```python
from build123d import *

# Parameters (mm, degrees)
F1_DEPTH = 130
F2_R     = 5.5
F3_DEPTH = 25
F2_R_2   = 9.5
F4_DEPTH = 13
F6_D     = 6.8
F7_D     = 8.8


# Not quite as in the source:
# - a pattern or mirror of a feature is missing from the dataset's text; its kind, count and spacing are read off the source's solid


with BuildPart() as f1:
    # F0 (on Front) → F1 (new body, symmetric)
    with BuildSketch(Plane.XZ):
        Polygon((-50, 23), (-50, 0), (45, 0), (45, -5), (50, -5), (50, 23), align=None)
    extrude(amount=F1_DEPTH, both=True)

    # F2 (on face) → F3 (cut)
    with BuildSketch(Plane.XY.offset(23)):
        with Locations((-36, -109)):
            Circle(F2_R)
        with Locations((36, -109)):
            Circle(F2_R)
        with Locations((-36, -57)):
            Circle(F2_R)
        with Locations((36, -57)):
            Circle(F2_R)
    f3 = extrude(amount=-F3_DEPTH, mode=Mode.SUBTRACT)

    # F3_copies: F3 across plane
    add(f3.mirror(Plane.ZX), mode=Mode.SUBTRACT)

    # F2 (on face) → F4 (cut)
    with BuildSketch(Plane.XY.offset(23)):
        with Locations((-36, -109)):
            Circle(F2_R_2)
        with Locations((-36, -109)):
            Circle(F2_R, mode=Mode.SUBTRACT)
        with Locations((36, -109)):
            Circle(F2_R_2)
        with Locations((36, -109)):
            Circle(F2_R, mode=Mode.SUBTRACT)
        with Locations((36, -109)):
            Circle(F2_R)
        with Locations((-36, -57)):
            Circle(F2_R_2)
        with Locations((-36, -57)):
            Circle(F2_R, mode=Mode.SUBTRACT)
        with Locations((36, -57)):
            Circle(F2_R_2)
        with Locations((36, -57)):
            Circle(F2_R, mode=Mode.SUBTRACT)
        with Locations((36, -57)):
            Circle(F2_R)
    f4 = extrude(amount=-F4_DEPTH, mode=Mode.SUBTRACT)

    # F4_copies: F4 across plane
    add(f4.mirror(Plane.ZX), mode=Mode.SUBTRACT)

    # F6 (through all)
    with Locations(Plane.XY.offset(23)):
        with Locations((-19, -115), (19, -115), (-19, -45), (19, -45), (19, -5), (-19, -5)):
            Hole(F6_D / 2)

    # F7 (through all)
    with Locations(Plane.XY.offset(23)):
        with Locations((-41, 35), (41, 35), (41, 90), (-41, 90)):
            Hole(F7_D / 2)


solid = f1.part
```
Can you work these out from the model? Positions are in its coordinate system, mm. A direction names the side the tool comes from. Round coordinates to 2 decimals unless told otherwise and drop trailing zeros. Order: outer loops, then holes, each group sorted by start corner. A loop starts at its lowest first (then second) coordinate and runs counter-clockwise, first axis right, second up.
(1) I'm going to push flat-ended pins straight in: pin 1 (3 mm diameter, centred on x = -0.5, y = -7.5, fed in from -Z); pin 2 (11.5 mm diameter, centred on x = -36, y = -57, fed in from +Z); pin 3 (4 mm diameter, centred on y = 111.5, z = -3, fed in from -X). Where does each tip first touch, or does it pass through?
Results are:
pin 1: stops at z = 0
pin 2: stops at z = 10
pin 3: stops at x = 45
(2) On a 3-axis mill with a long thin cutter (end or side, diameter ignored), from which of +Z, -Z, +X, -X, +Y, -Y can I reach the whole of each face in a straight line? I mean faces 5 (the face through (19.44, -41.63, 11.34)), 6 (the face through (-26.939, 106.146, 16.591)). Say none if no direction works.
Results are:
face 5: +Z, -Z
face 6: +Z
(3) If I drill on L1, parallel to Y at x = -35, z = 18; L2, parallel to Y at x = -36, z = 3.75; L3, parallel to Y at x = 19, z = 6, over which ranges is the centre line in solid material (lowest first)?
Results are:
L1: y = -130 to -118.45, -99.55 to -66.45, -47.55 to 47.55, 66.45 to 99.55, 118.45 to 130
L2: y = -130 to -114.5, -103.5 to -62.5, -51.5 to 51.5, 62.5 to 103.5, 114.5 to 130
L3: y = -130 to -118.4, -111.6 to -48.4, -41.6 to -8.4, -1.6 to 130
(4) If we section it at C-C (y = -76): Please give me the cut outline in (x, z).
Results are:
outline: (-50, 0) - (45, 0) - (45, -5) - (50, -5) - (50, 23) - (-50, 23) - close
(5) If we section it at D-D (x = 1): Please give me the cut outline in (y, z).
Results are:
outline: (-130, 0) - (130, 0) - (130, 23) - (-130, 23) - close
(6) If we section it at B-B (z = 19.75): Count the separate pieces of the cut face and the enclosed holes in it, plus the area to 3 significant figures.
Results are:
separate pieces: 1
enclosed holes: 18
area: 23,300 mm2
(7) If we section it at A-A (y = 57): Please give me the cut outline in (x, z), plus the area to 3 significant figures.
Results are:
outline: (-50, 0) - (-41.5, 0) - (-41.5, 10) - (-45.5, 10) - (-45.5, 23) - (-50, 23) - close; (-30.5, 0) - (30.5, 0) - (30.5, 10) - (26.5, 10) - (26.5, 23) - (-26.5, 23) - (-26.5, 10) - (-30.5, 10) - close; (41.5, 0) - (45, 0) - (45, -5) - (50, -5) - (50, 23) - (45.5, 23) - (45.5, 10) - (41.5, 10) - close
area: 1,610 mm2
(8) We'd pull the mould along X, two halves only. Please class faces 1 (the face through (-1, -130, 12)), 2 (the face through (50, -2, 9)), 3 (the face through (-41.495, 56.758, 5.07)), 4 (the face through (45, -50, -2)): +X half, -X half, draft (parallel to the pull), parting line (faces both ways), or undercut.
Results are:
face 1: draft
face 2: +X half
face 3: undercut
face 4: -X half
